from build123d import *

# Parameters (mm, degrees)
SKETCH1_W           = 339
SKETCH1_H           = 253
BOSS_EXTRUDE1_DEPTH = 150
SHELL1_T            = -3
SKETCH2_R           = 6


with BuildPart() as part:
    # Sketch1 → Boss-Extrude1 (new body)
    with BuildSketch(Plane(origin=(0, 0, 0), x_dir=(1, 0, 0), z_dir=(0, 1, 0))):
        with Locations((-6.320083682, -6.625523013)):
            Rectangle(SKETCH1_W, SKETCH1_H)
    extrude(amount=BOSS_EXTRUDE1_DEPTH)

    # Shell1
    shell1_openings = [part.faces().sort_by_distance(p)[0] for p in [
        (-6.320083682, 150, 6.625523013),
    ]]
    offset(amount=SHELL1_T, openings=shell1_openings, kind=Kind.INTERSECTION)

    # Sweep2: sweep along a path in Sketch4
    with BuildLine(Plane(origin=(0, 83.172395684, 0), x_dir=(1, 0, 0), z_dir=(0, 1, 0))) as sweep2_path:
        Line((163.179916318, -68.125523013), (169.565605174, -68.125523013))
        ThreePointArc((169.565605174, -68.125523013), (176.636672985, -65.196590824), (179.565605174, -58.125523013))
        Line((179.565605174, -58.125523013), (179.565605174, 44.874476987))
        ThreePointArc((179.565605174, 44.874476987), (176.636672985, 51.945544799), (169.565605174, 54.874476987))
        Line((169.565605174, 54.874476987), (163.179916318, 54.874476987))
    # Sketch2 → Sweep2 (sweep)
    with BuildSketch(Plane(origin=(163.179916318, 0, 0), x_dir=(0, 0, -1), z_dir=(1, 0, 0))):
        with Locations((-68.125523013, 83.172395684)):
            Circle(SKETCH2_R)
    sweep(path=sweep2_path.line)


solid = part.part
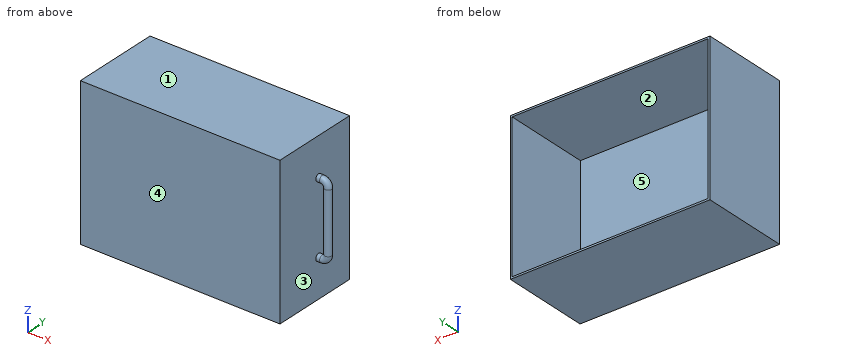
The listing builds one solid part. Answer for the finished solid, in the listing's coordinates (mm). Face numbers are marked on the shaded views. A direction names the side the tool comes from. Round coordinates to 2 decimals unless told otherwise and drop trailing zeros. Order: outer loops, then holes, each group sorted by start corner. A loop starts at its lowest first (then second) coordinate and runs counter-clockwise, first axis right, second up. Notation, with made-up numbers: (29.25, -27) -> (58.25, -27) arc R29 cw to (58.25, -2) -> close; hole circle Ø7 at (64, 3.25). An arc over 180 degrees is marked (long way). One line per item, written item: value.
Item 1: For a pull along Y with two mould halves and no side action, classify the marked faces 3, 4 and 5 as released by +Y, released by -Y, zero draft, split by the parting line, or undercut.
Taken from the geometry:
face 3: zero draft
face 4: released by -Y
face 5: released by +Y
Item 2: Find section C-C, the plane z = -65.5. Give the vertices of the cut face in (x, y).
Taken from the geometry:
outline: (-175.82, 0) -> (163.18, 0) -> (163.18, 150) -> (160.18, 150) -> (160.18, 3) -> (-172.82, 3) -> (-172.82, 150) -> (-175.82, 150) -> close
Item 3: For the marked faces 1 and 2, determine the directions among +Z, -Z, +X, -X, +Y, -Y from which every point of the face is accessible in a straight line to the end or side of a thin tool.
Taken from the geometry:
face 1: +Z, +X, -X, +Y, -Y
face 2: +Y
Item 4: Find section D-D, the plane z = 6.5. Give the vertices of the cut face in (x, y), then the cut area to 3 significant figures.
Taken from the geometry:
outline: (-175.82, 0) -> (163.18, 0) -> (163.18, 150) -> (160.18, 150) -> (160.18, 3) -> (-172.82, 3) -> (-172.82, 150) -> (-175.82, 150) -> close; circle Ø12 at (179.57, 83.17)
area: 2,010 mm2
Item 5: Given P1, Ø8, axis at y = 101.5, z = -77.5, coming from the +X side; P2, Ø8, axis at x = 74, z = -32.5, coming from the +Y side, each flat-ended and moving along its own axis, determine where each tip first touches the part or whether it passes through.
Taken from the geometry:
P1: stops at x = 163.18
P2: stops at y = 3
Item 6: Find section A-A, the plane y = 16.5. Give the vertices of the cut face in (x, z), then the cut area to 3 significant figures.
Taken from the geometry:
outline: (-175.82, -119.87) -> (163.18, -119.87) -> (163.18, 133.13) -> (-175.82, 133.13) -> close; hole (-172.82, -116.87) -> (160.18, -116.87) -> (160.18, 130.13) -> (-172.82, 130.13) -> close
area: 3,520 mm2
Item 7: Straight lines are drawn through the part: L1, parallel to X at y = 132, z = -78.5; L2, parallel to Z at x = -142.5, y = 78.5; L3, parallel to Y at x = 131.5, z = 11. For each, find the intervals that lie inside material, in ascending order.
Taken from the geometry:
L1: x = -175.82 to -172.82, 160.18 to 163.18
L2: z = -119.87 to -116.87, 130.13 to 133.13
L3: y = 0 to 3
Item 8: Find section B-B, the plane x = 124. Give the vertices of the cut face in (y, z).
Taken from the geometry:
outline: (0, -119.87) -> (150, -119.87) -> (150, -116.87) -> (3, -116.87) -> (3, 130.13) -> (150, 130.13) -> (150, 133.13) -> (0, 133.13) -> close
